The listing builds one solid part. Answer for the finished solid, in the listing's coordinates (mm). A direction names the side the tool comes from. Give positions to 0.01 mm unless a question says otherwise; leave off trailing zeros. Write each loop counter-clockwise with the first axis right and the second up, starting at its lowest first coordinate (ties: lowest second). Pieces come first, ordered by that corner, then holes. Notation, with made-up numbers: (22, -8.5) -> (59, -8.5) arc R11 cw to (59, -4.5) -> close; hole circle Ø5 at (0, 81). An arc over 180 degrees is marked (long way). One line per question, with ' | ' between items.
from build123d import *

# Parameters (mm, degrees)
BOSS_EXTRUDE1_DEPTH      = 55.5
BOSS_EXTRUDE1_DEPTH_BACK = 55.5
SKETCH2_R                = 45
BOSS_EXTRUDE2_DEPTH      = 10
FILLET1_R                = 3


with BuildPart() as part:
    # Sketch1 → Boss-Extrude1 (new body, two sides)
    with BuildSketch(Plane(origin=(0, 0, 0), x_dir=(1, 0, 0), z_dir=(0, 1, 0))) as boss_extrude1_sk:
        with BuildLine():
            Line((0, 0), (65, 0))
            Line((65, 0), (150.7127313, 47.511342784))
            Line((150.7127313, 47.511342784), (153.155696069, 117.468700675))
            Line((153.155696069, 117.468700675), (107.256349668, 143.968700675))
            ThreePointArc((107.256349668, 143.968700675), (79.846161337, 150.2914933), (53.590163022, 140.196014935))
            Line((53.590163022, 140.196014935), (15, 110))
            Line((15, 110), (0, 110))
            Line((0, 110), (0, 0))
        make_face()
    extrude(amount=BOSS_EXTRUDE1_DEPTH)
    extrude(boss_extrude1_sk.sketch, amount=-BOSS_EXTRUDE1_DEPTH_BACK)

    # Sketch2 → Boss-Extrude2 (add)
    with BuildSketch(Plane.ZY):
        with Locations((-55, 0)):
            Circle(SKETCH2_R)
    extrude(amount=BOSS_EXTRUDE2_DEPTH)

    # Fillet1
    fillet1_edges = [part.edges().sort_by_distance(p)[0] for p in [
        (0, 0, -100),
    ]]
    fillet(fillet1_edges, radius=FILLET1_R)


with BuildPart() as part_1:
    # Body-Move_Copy1: moved
    add(part.part.moved(Location((-83.217640918, 0, 55))))


solid = part_1.part
Item 1: A tool of negligible diameter and unlimited length cuts with its end or side. For faces 1 (the face through (-8, -55.5, -21)), 2 (the face through (-83.218, 1, -50)), 3 (the face through (-76, 1, -55)), from which of +Z, -Z, +X, -X, +Y, -Y can it reach the whole face along a straight path? Write none if from no direction.
Answers below:
face 1: +Z, -Z, +X, -X, -Y | face 2: -X | face 3: -Z, -X, +Y, -Y
Item 2: Consider line 1 (X direction, y = -44, z = 17); line 2 (Z direction, x = -18, y = -49); line 3 (X direction, y = 11, z = 11.5). Determine where each line is inside the solid, lowest interval first. Write a range as [from, to].
Answers below:
line 1: [-83.33, 50.34] | line 2: [-91.91, 54.88] | line 3: [-93.22, 60.26]
Item 3: Flat-ended cylindrical pins translate along their axes: pin 1 (2 mm diameter, centred on x = 9.5, y = -0.5, fed in from -Z); pin 2 (1 mm diameter, centred on y = -20, z = 27.5, fed in from +X); pin 3 (1.5 mm diameter, centred on x = -48, y = 26.5, fed in from -Z). Find the tip coordinate at first contact, or state that the pin passes through.
Answers below:
pin 1: z = -94.65 | pin 2: x = 32.3 | pin 3: z = -71.41
Item 4: Find section C-C (x = 20.5). Write down the section's boundary in (y, z).
Answers below:
outline: (-55.5, -90.82) -> (55.5, -90.82) -> (55.5, 33.54) -> (-55.5, 33.54) -> close
Item 5: Find section B-B (z = 0). Write down the section's boundary in (x, y).
Answers below:
outline: (-93.22, -45) -> (-86.22, -45) arc R3 cw to (-83.22, -48) -> (-83.22, -55.5) -> (67.76, -55.5) -> (67.76, 55.5) -> (-83.22, 55.5) -> (-83.22, 48) arc R3 cw to (-86.22, 45) -> (-93.22, 45) -> close
Item 6: Find section A-A (y = 0). Write down the section's boundary in (x, z), then the cut area to 3 significant figures.
Answers below:
outline: (-93.22, -45) -> (-86.22, -45) arc R3 cw to (-83.22, -48) -> (-83.22, -55) -> (-68.22, -55) -> (-29.63, -85.2) arc R48.08 ccw to (24.04, -88.97) -> (69.94, -62.47) -> (67.5, 7.49) -> (-18.22, 55) -> (-83.22, 55) -> (-83.22, 48) arc R3 cw to (-86.22, 45) -> (-93.22, 45) -> close | area: 19,100 mm²
Item 7: Find section D-D (z = -71.5). Write down the section's boundary in (x, y).
Answers below:
outline: (-47.13, -55.5) -> (54.3, -55.5) -> (54.3, 55.5) -> (-47.13, 55.5) -> close
